Can you work these out from the drawing? Everything is in mm from the part's minimum corner. Give positions to 0.01 mm unless a question says otherwise; leave off trailing zeros. Loops run counter-clockwise (first coordinate to the right, second up) from the corner with the lowest first, then second, coordinate; pieces in that order, holes last. Notation, with made-up numbers: (24.25, -39) -> (79.25, -39) arc R9 cw to (79.25, -27) -> close; hole circle Ø3 at (-20.75, 44.25). An arc over 180 degrees is marked (long way). Write item = value, one per line. Start each with the question number.
1) I want a section at C-C (x = 6.5). List the corners of the cut face in (y, z) for me.
2) I want a section at A-A (z = 4). List the corners of the cut face in (x, y) for me.
3) I need wall thicknesses on probe 1 along Z at (x, y) = (4, 3); probe 2 along Z at (x, y) = (5, 5); probe 3 along X at (y, z) = (3, 3.5). Which ranges of each line are inside material? Lowest first, please. Write a range as from..to.
4) I want a section at B-B (y = 6.5). List the corners of the cut face in (x, z) for me, and give its area (3 significant figures).
5) I'm going to push a flat-ended pin straight in: pin 1 Ø3.5 at (x, z) = (4, 4) entering from +Y. Where does the tip first touch, or does it pass through?
6) I want a section at D-D (z = 5.5). List the corners of the cut face in (x, y) for me.
7) If we mould it in two halves opening along X, with no side actions, what happens to the marked faces 1, 2, 3 and 4? For each: +X half, -X half, draft (parallel to the pull), parting line (faces both ways), or undercut.
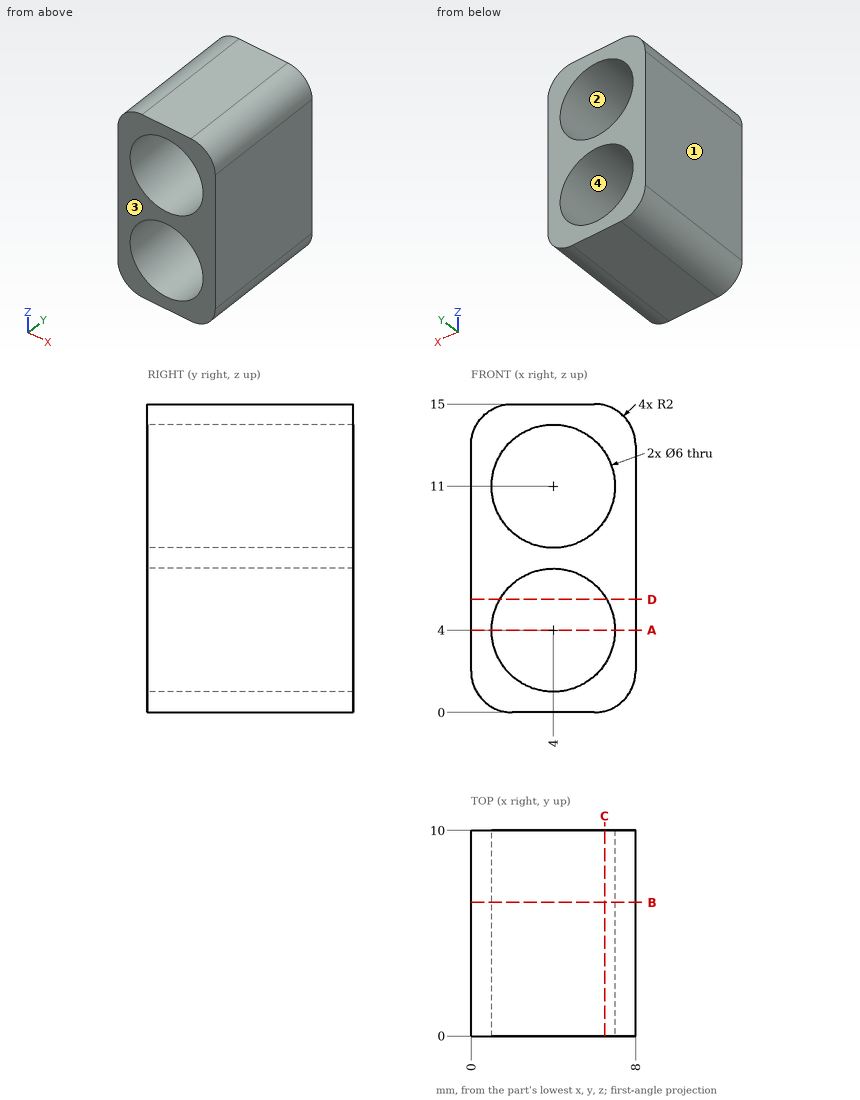
Answer list:
q1.outline = (0, 0.06) -> (10, 0.06) -> (10, 2.34) -> (0, 2.34) -> close; (0, 5.66) -> (10, 5.66) -> (10, 9.34) -> (0, 9.34) -> close; (0, 12.66) -> (10, 12.66) -> (10, 14.94) -> (0, 14.94) -> close
q2.outline = (0, 0) -> (1, 0) -> (1, 10) -> (0, 10) -> close; (7, 0) -> (8, 0) -> (8, 10) -> (7, 10) -> close
q3.probe_1 = 0..1, 7..8, 14..15
q3.probe_2 = 0..1.17, 6.83..8.17, 13.83..15
q3.probe_3 = 0..1.04, 6.96..8
q4.outline = (0, 2) arc R2 ccw to (2, 0) -> (6, 0) arc R2 ccw to (8, 2) -> (8, 13) arc R2 ccw to (6, 15) -> (2, 15) arc R2 ccw to (0, 13) -> close; hole circle Ø6 at (4, 4); hole circle Ø6 at (4, 11)
q4.area = 60.0 mm^2
q5.pin_1 = through
q6.outline = (0, 0) -> (1.4, 0) -> (1.4, 10) -> (0, 10) -> close; (6.6, 0) -> (8, 0) -> (8, 10) -> (6.6, 10) -> close
q7.face_1 = -X half
q7.face_2 = undercut
q7.face_3 = draft
q7.face_4 = undercut
